from build123d import *

# Parameters (mm, degrees)
F1_DEPTH = 60
F2_R     = 12.5
F3_DEPTH = 99
F4_SIZE  = 5
F5_SIZE  = 5
F6_SIZE  = 5
F7_SIZE  = 5


with BuildPart() as f1:
    # F0 (on Front) → F1 (new body)
    with BuildSketch(Plane.XZ):
        Polygon((-7.1532973647, 28.6979936063), (-67.1532973647, 28.6979936063), (-67.1532973647, -31.3020063937), (132.8467026353, -31.3020063937), (132.8467026353, 28.6979936063), (72.8467026353, 28.6979936063), (72.8467026353, -11.3020063937), (-7.1532973647, -11.3020063937), align=None)
    extrude(amount=F1_DEPTH)

    # F2 (on face) → F3 (cut)
    with BuildSketch(Plane.YZ.offset(132.8467026353)):
        with Locations((-30, 8.6979936063)):
            Circle(F2_R)
    extrude(amount=-F3_DEPTH, mode=Mode.SUBTRACT)

    # F4
    f4_edges = [f1.edges().sort_by_distance(p)[0] for p in [
        (-67.153297, -60, -1.302006),
        (-67.153297, 0, -1.302006),
    ]]
    chamfer(f4_edges, length=F4_SIZE)

    # F5 (call 1 of 2: OpenCascade refuses the feature's edges together)
    f5_edges = [f1.edges().sort_by_distance(p)[0] for p in [
        (35.346703, -60, -31.302006),
    ]]
    chamfer(f5_edges, length=F5_SIZE)

    # F5#2 (call 2 of 2)
    f5_2_edges = [f1.edges().sort_by_distance(p)[0] for p in [
        (-67.153297, -30, -31.302006),
    ]]
    chamfer(f5_2_edges, length=F5_SIZE)

    # F6
    f6_edges = [f1.edges().sort_by_distance(p)[0] for p in [
        (-67.153297, -30, 28.697994),
        (132.846703, -30, 28.697994),
        (102.846703, 0, 28.697994),
        (102.846703, -60, 28.697994),
        (72.846703, -30, 28.697994),
        (35.346703, 0, -31.302006),
    ]]
    chamfer(f6_edges, length=F6_SIZE)

    # F7 (call 1 of 4: OpenCascade refuses the feature's edges together)
    f7_edges = [f1.edges().sort_by_distance(p)[0] for p in [
        (132.846703, -60, -1.302006),
    ]]
    chamfer(f7_edges, length=F7_SIZE)

    # F7#2 (call 2 of 4)
    f7_2_edges = [f1.edges().sort_by_distance(p)[0] for p in [
        (132.846703, 0, -1.302006),
    ]]
    chamfer(f7_2_edges, length=F7_SIZE)

    # F7#3 (call 3 of 4)
    f7_3_edges = [f1.edges().sort_by_distance(p)[0] for p in [
        (132.846703, -30, -31.302006),
    ]]
    chamfer(f7_3_edges, length=F7_SIZE)

    # F7#4 (call 4 of 4)
    f7_4_edges = [f1.edges().sort_by_distance(p)[0] for p in [
        (-7.153297, -30, 28.697994),
        (-34.653297, -60, 28.697994),
        (-34.653297, 0, 28.697994),
    ]]
    chamfer(f7_4_edges, length=F7_SIZE)


solid = f1.part
Design review of the part built by this model. Coordinates are the model's own, in mm. A direction names the side the tool comes from. Coordinates: 2 decimals unless noted, no trailing zeros. Order: outer loops, then holes, each group sorted by start corner. A loop starts at its lowest first (then second) coordinate and runs counter-clockwise, first axis right, second up. Notation, with made-up numbers: (-16, -31.5) -> (33, -31.5) arc R23 ccw to (33, -22.5) -> close; hole circle Ø7 at (50, 72). An arc over 180 degrees is marked (long way). Use one line per item in the form item = value. Start each with the question number.
(1) For faces 1 (the flat face through (-64.618, -29.615, -28.837)), 2 (the flat face through (75.31, -29.58, 26.16)), list the 3-axis set-ups (+Z, -Z, +X, -X, +Y, -Y) from which the entire face can be reached by the end or side of a thin tool; tool diameter is ignored.
(2) Insertion check: pin 1 (12 mm diameter, centred on x = 39, y = -14, fed in from +Z); pin 2 (22.5 mm diameter, centred on y = -30, z = 8.7, fed in from +X). Each pin has a flat end and moves straight along its axis. Give the tip position at first contact, or say it passes through.
(3) For probe 1 along Z at (x, y) = (90.5, -30); probe 2 along X at (y, z) = (-9, 2.5); probe 3 along X at (y, z) = (-33, 9), list the stretches that pass through material, from the lowest coordinate up.
(4) Add section A-A on y = -30. State the section outline as (x, z) points.
(5) Add section B-B on y = -14.5. State the section outline as (x, z) points.
(6) Add section D-D on x = 58.5. State the section outline as (y, z) points.
(7) Add section C-C on z = 14.5. State the section outline as (x, y) points, plus the area to 3 significant figures.
(8) The part is to be moulded in two halves that separate along X. For faces 3 (the flat face through (72.847, -30, -5)), 4 (the flat face through (-67.153, -30, -1)), 5 (the flat face through (32, -60, -12)), say which applies: +X half, -X half, draft (parallel to the pull), parting line (faces both ways), or undercut.
Answer block:
q1.face_1 = -Z, -X, +Y, -Y
q1.face_2 = +Z, +Y, -Y
q2.pin_1 = -11.3
q2.pin_2 = -7.15
q3.probe_1 = -31.3 to -3.8, 21.2 to 28.7
q3.probe_2 = -67.15 to -7.15, 72.85 to 132.85
q3.probe_3 = -67.15 to -7.15
q4.outline = (-67.15, -26.3) -> (-62.15, -31.3) -> (127.85, -31.3) -> (132.85, -26.3) -> (132.85, -3.8) -> (72.85, -3.8) -> (72.85, -11.3) -> (-7.15, -11.3) -> (-7.15, 23.7) -> (-12.15, 28.7) -> (-62.15, 28.7) -> (-67.15, 23.7) -> close; (72.85, 21.2) -> (132.85, 21.2) -> (132.85, 23.7) -> (127.85, 28.7) -> (77.85, 28.7) -> (72.85, 23.7) -> close
q5.outline = (-67.15, -26.3) -> (-62.15, -31.3) -> (127.85, -31.3) -> (132.85, -26.3) -> (132.85, 23.7) -> (127.85, 28.7) -> (77.85, 28.7) -> (72.85, 23.7) -> (72.85, -11.3) -> (-7.15, -11.3) -> (-7.15, 23.7) -> (-12.15, 28.7) -> (-62.15, 28.7) -> (-67.15, 23.7) -> close
q6.outline = (-60, -26.3) -> (-55, -31.3) -> (-5, -31.3) -> (0, -26.3) -> (0, -11.3) -> (-60, -11.3) -> close
q7.outline = (-67.15, -55) -> (-62.15, -60) -> (-7.15, -60) -> (-7.15, 0) -> (-62.15, 0) -> (-67.15, -5) -> close; (72.85, -60) -> (127.85, -60) -> (132.85, -55) -> (132.85, -41.07) -> (72.85, -41.07) -> close; (72.85, -18.93) -> (132.85, -18.93) -> (132.85, -5) -> (127.85, 0) -> (72.85, 0) -> close
q7.area = 5,820 mm²
q8.face_3 = undercut
q8.face_4 = -X half
q8.face_5 = draft
